from build123d import *

# Parameters (mm, degrees)
SKETCH_W        = 114
SKETCH_H        = 92
SKETCH_R        = 3
PAD_DEPTH       = 2
SKETCH001_W     = 114
SKETCH001_H     = 92
SKETCH001_W_2   = 110
SKETCH001_H_2   = 88
PAD001_DEPTH    = 13
SKETCH003_W     = 59
SKETCH003_H     = 10
POCKET_DEPTH    = 5
SKETCH004_W     = 11
SKETCH004_H     = 6.2
POCKET001_DEPTH = 5
SKETCH005_W     = 21
SKETCH005_H     = 21
POCKET002_DEPTH = 5
SKETCH006_W     = 9.2
SKETCH006_H     = 11
POCKET003_DEPTH = 5
FILLET_R        = 0.5


with BuildPart() as part:
    # Sketch → Pad (new body)
    with BuildSketch(Plane.XY):
        Rectangle(SKETCH_W, SKETCH_H)
        with Locations((-46, 23.5)):
            Circle(SKETCH_R, mode=Mode.SUBTRACT)
        with Locations((46, -17.5)):
            Circle(SKETCH_R, mode=Mode.SUBTRACT)
    extrude(amount=PAD_DEPTH)

    # Sketch001 (on Face8 of Pad) → Pad001 (join)
    with BuildSketch(Plane.XY.offset(2)):
        Rectangle(SKETCH001_W, SKETCH001_H)
        Rectangle(SKETCH001_W_2, SKETCH001_H_2, mode=Mode.SUBTRACT)
    extrude(amount=PAD001_DEPTH)

    # Sketch003 (on Face12 of Pad001) → Pocket (cut)
    with BuildSketch(Plane.XZ.offset(46)):
        with Locations((0, 15.6)):
            Rectangle(SKETCH003_W, SKETCH003_H)
    extrude(amount=-POCKET_DEPTH, mode=Mode.SUBTRACT)

    # Sketch004 (on Face5 of Pocket) → Pocket001 (cut)
    with BuildSketch(Plane(origin=(0, 46, 0), x_dir=(-1, 0, 0), z_dir=(0, 1, 0))):
        with Locations((0, 12.1)):
            Rectangle(SKETCH004_W, SKETCH004_H)
    extrude(amount=-POCKET001_DEPTH, mode=Mode.SUBTRACT)

    # Sketch005 (on Face5 of Pocket001) → Pocket002 (cut)
    with BuildSketch(Plane(origin=(0, 46, 0), x_dir=(-1, 0, 0), z_dir=(0, 1, 0))):
        with Locations((30.48, 21.1)):
            Rectangle(SKETCH005_W, SKETCH005_H)
    extrude(amount=-POCKET002_DEPTH, mode=Mode.SUBTRACT)

    # Sketch006 (on Face5 of Pocket002) → Pocket003 (cut)
    with BuildSketch(Plane(origin=(0, 46, 0), x_dir=(-1, 0, 0), z_dir=(0, 1, 0))):
        with Locations((-33, 16.1)):
            Rectangle(SKETCH006_W, SKETCH006_H)
    extrude(amount=-POCKET003_DEPTH, mode=Mode.SUBTRACT)

    # Fillet
    fillet_edges = [part.edges().sort_by_distance(p)[0] for p in [
        (-57, 46, 1),
        (57, 46, 1),
        (0, 46, 0),
        (-57, -46, 1),
        (-57, 0, 0),
        (57, -46, 1),
        (57, 0, 0),
        (0, -46, 0),
        (43, -17.5, 0),
        (-49, 23.5, 0),
        (57, 46, 8.5),
        (37.6, 46, 12.8),
        (33, 46, 10.6),
        (28.4, 46, 12.8),
        (5.5, 46, 12),
        (0, 46, 9),
        (-5.5, 46, 12),
        (-19.98, 46, 12.8),
        (-40.98, 46, 12.8),
        (-48.99, 46, 15),
        (-57, 46, 8.5),
        (37.6, 45, 10.6),
        (28.4, 45, 10.6),
        (5.5, 45, 9),
        (-19.98, 45, 10.6),
        (-30.48, 46, 10.6),
        (-40.98, 45, 10.6),
        (57, -46, 8.5),
        (-57, -46, 8.5),
        (0, -46, 10.6),
        (29.5, -46, 12.8),
        (-29.5, -45, 10.6),
        (-29.5, -46, 12.8),
        (-29.5, -44, 12.8),
        (0, 44, 2),
        (55, 0, 2),
        (0, -44, 2),
        (-5.5, 45, 9),
    ]]
    fillet(fillet_edges, radius=FILLET_R)


solid = part.part
Build history of the part. All positions in model axes, mm. A direction names the side the tool comes from. Round coordinates to 2 decimals unless told otherwise and drop trailing zeros. Write each loop counter-clockwise with the first axis right and the second up, starting at its lowest first coordinate (ties: lowest second). Pieces come first, ordered by that corner, then holes. Notation, with made-up numbers: (-23, -7) -> (35, -7) arc R21 cw to (35, 30) -> close; hole circle Ø4 at (-39, 77.25). An arc over 180 degrees is marked (long way). Use one line per item in the form item = value.
Q1. Tool access for faces 4 (the flat face through (-57, -1, 8)), 5 (the flat face through (-1, 44, 7)): list every direction of +Z, -Z, +X, -X, +Y, -Y with a clear straight run to the whole face (end or side of a thin tool).
Conclusion:
face_4 = +Z, -Z, -X, +Y, -Y
face_5 = +Z
Q2. Drop flat-ended pins along their axis: P1, Ø3, axis at x = -36.5, y = -19, coming from the -Z side; P2, Ø2, axis at x = -9.5, z = 13, coming from the -Y side; P3, Ø12, axis at x = 41, y = -6.5, coming from the +Z side. Give the stop position or say it passes through.
Conclusion:
P1 = 0
P2 = 44
P3 = 2
Q3. Band-saw the part on D-D, the plane y = -2. Write the cut outline in (x, z), then the cut area to 3 significant figures.
Conclusion:
outline = (-57, 0.5) arc R0.5 ccw to (-56.5, 0) -> (56.5, 0) arc R0.5 ccw to (57, 0.5) -> (57, 15) -> (55, 15) -> (55, 2.5) arc R0.5 cw to (54.5, 2) -> (-55, 2) -> (-55, 15) -> (-57, 15) -> close
area = 280 mm²
Q4. Band-saw the part on C-C, the plane z = 4.5. Write the cut outline in (x, y).
Conclusion:
outline = (-57, -45.5) arc R0.5 ccw to (-56.5, -46) -> (56.5, -46) arc R0.5 ccw to (57, -45.5) -> (57, 45.5) arc R0.5 ccw to (56.5, 46) -> (-56.5, 46) arc R0.5 ccw to (-57, 45.5) -> close; hole (-55, -44) -> (55, -44) -> (55, 44) -> (-55, 44) -> close
Q5. Drill centre lines: L1, parallel to Y at x = 46, z = 1.6; L2, parallel to Y at x = -46, z = 1.25; L3, parallel to X at y = 24, z = 11. Where is each one in solid material? Low to high.
Conclusion:
L1 = -46 to -20.5, -14.5 to 46
L2 = -46 to 20.5, 26.5 to 46
L3 = -57 to -55, 55 to 57
Q6. Band-saw the part on A-A, the plane x = 46. Write the cut outline in (y, z), then the cut area to 3 significant figures.
Conclusion:
outline = (-46, 0.5) arc R0.5 ccw to (-45.5, 0) -> (-21, 0) arc R0.5 ccw to (-20.5, 0.5) -> (-20.5, 2) -> (-43.5, 2) arc R0.5 cw to (-44, 2.5) -> (-44, 15) -> (-46, 15) -> close; (-14.5, 0.5) arc R0.5 ccw to (-14, 0) -> (45.5, 0) arc R0.5 ccw to (46, 0.5) -> (46, 15) -> (44, 15) -> (44, 2.5) arc R0.5 cw to (43.5, 2) -> (-14.5, 2) -> close
area = 224 mm²
Q7. Two-plate mould, pull along X, no slides. Class faces 1 (the flat face through (-1, 1, 0)), 2 (the cylindrical face through (43.6, -19.3, 1.2)), 3 (the flat face through (57, -1, 8)): released by +X, released by -X, zero draft, split by the parting line, or undercut.
Conclusion:
face_1 = zero draft
face_2 = undercut
face_3 = released by +X
Q8. Band-saw the part on B-B, the plane y = -17.5. Write the cut outline in (x, z).
Conclusion:
outline = (-57, 0.5) arc R0.5 ccw to (-56.5, 0) -> (42.5, 0) arc R0.5 ccw to (43, 0.5) -> (43, 2) -> (-55, 2) -> (-55, 15) -> (-57, 15) -> close; (49, 0.5) arc R0.5 ccw to (49.5, 0) -> (56.5, 0) arc R0.5 ccw to (57, 0.5) -> (57, 15) -> (55, 15) -> (55, 2.5) arc R0.5 cw to (54.5, 2) -> (49, 2) -> close
